```python
from build123d import *

# Parameters (mm, degrees)
EXTRUDE_1_DEPTH     = 8
SKETCH_2_W          = 51
SKETCH_2_H          = 5
EXTRUDE_2_DEPTH     = 28.7
SKETCH_3_R          = 17.5
CUT_EXTRUDE_1_DEPTH = 2
CUT_EXTRUDE_2_REACH = 82.708
SKETCH_4_R          = 1.25
SKETCH_5_R          = 1.5
CUT_EXTRUDE_3_DEPTH = 5


with BuildPart() as part:
    # 스케치1 → 보스-돌출1 (new body)
    with BuildSketch(Plane.XY):
        with BuildLine():
            Line((0, 0), (0, 54.5))
            Line((0, 54.5), (51, 54.5))
            Line((51, 54.5), (51, 0))
            ThreePointArc((51, 0), (25.5, -25.5), (0, 0))
        make_face()
    extrude(amount=EXTRUDE_1_DEPTH)

    # 스케치2 → 보스-돌출2 (add)
    with BuildSketch(Plane(origin=(0, 0, 0), x_dir=(-1, 0, 0), z_dir=(0, 0, -1))):
        with Locations((-25.5, 52)):
            Rectangle(SKETCH_2_W, SKETCH_2_H)
    extrude(amount=EXTRUDE_2_DEPTH)

    # 스케치3 → 컷-돌출1 (cut)
    with BuildSketch(Plane(origin=(0, 0, 0), x_dir=(-1, 0, 0), z_dir=(0, 0, -1))):
        with Locations((-25.5, 0)):
            Circle(SKETCH_3_R)
    extrude(amount=-CUT_EXTRUDE_1_DEPTH, mode=Mode.SUBTRACT)

    # 스케치4 → 컷-돌출2 (cut, up to next)
    with BuildSketch(Plane(origin=(0, 0, 2), x_dir=(-1, 0, 0), z_dir=(0, 0, -1)), mode=Mode.PRIVATE) as cut_extrude_2_sk1:
        with Locations((-25.5, 13.75)):
            Circle(SKETCH_4_R)
    cut_extrude_2_tool1 = extrude(cut_extrude_2_sk1.sketch, amount=-CUT_EXTRUDE_2_REACH, mode=Mode.PRIVATE) & part.part
    # 스케치4 → 컷-돌출2 (cut, up to next)
    with BuildSketch(Plane(origin=(0, 0, 2), x_dir=(-1, 0, 0), z_dir=(0, 0, -1)), mode=Mode.PRIVATE) as cut_extrude_2_sk2:
        with Locations((-13.592150698, 6.875)):
            Circle(SKETCH_4_R)
    cut_extrude_2_tool2 = extrude(cut_extrude_2_sk2.sketch, amount=-CUT_EXTRUDE_2_REACH, mode=Mode.PRIVATE) & part.part
    # 스케치4 → 컷-돌출2 (cut, up to next)
    with BuildSketch(Plane(origin=(0, 0, 2), x_dir=(-1, 0, 0), z_dir=(0, 0, -1)), mode=Mode.PRIVATE) as cut_extrude_2_sk3:
        with Locations((-13.592150698, -6.875)):
            Circle(SKETCH_4_R)
    cut_extrude_2_tool3 = extrude(cut_extrude_2_sk3.sketch, amount=-CUT_EXTRUDE_2_REACH, mode=Mode.PRIVATE) & part.part
    # 스케치4 → 컷-돌출2 (cut, up to next)
    with BuildSketch(Plane(origin=(0, 0, 2), x_dir=(-1, 0, 0), z_dir=(0, 0, -1)), mode=Mode.PRIVATE) as cut_extrude_2_sk4:
        with Locations((-25.5, -13.75)):
            Circle(SKETCH_4_R)
    cut_extrude_2_tool4 = extrude(cut_extrude_2_sk4.sketch, amount=-CUT_EXTRUDE_2_REACH, mode=Mode.PRIVATE) & part.part
    # 스케치4 → 컷-돌출2 (cut, up to next)
    with BuildSketch(Plane(origin=(0, 0, 2), x_dir=(-1, 0, 0), z_dir=(0, 0, -1)), mode=Mode.PRIVATE) as cut_extrude_2_sk5:
        with Locations((-37.407849302, -6.875)):
            Circle(SKETCH_4_R)
    cut_extrude_2_tool5 = extrude(cut_extrude_2_sk5.sketch, amount=-CUT_EXTRUDE_2_REACH, mode=Mode.PRIVATE) & part.part
    # 스케치4 → 컷-돌출2 (cut, up to next)
    with BuildSketch(Plane(origin=(0, 0, 2), x_dir=(-1, 0, 0), z_dir=(0, 0, -1)), mode=Mode.PRIVATE) as cut_extrude_2_sk6:
        with Locations((-37.407849302, 6.875)):
            Circle(SKETCH_4_R)
    cut_extrude_2_tool6 = extrude(cut_extrude_2_sk6.sketch, amount=-CUT_EXTRUDE_2_REACH, mode=Mode.PRIVATE) & part.part
    add(cut_extrude_2_tool1.solids().sort_by_distance((25.5, 13.75, 2))[0], mode=Mode.SUBTRACT)
    add(cut_extrude_2_tool2.solids().sort_by_distance((13.592151, 6.875, 2))[0], mode=Mode.SUBTRACT)
    add(cut_extrude_2_tool3.solids().sort_by_distance((13.592151, -6.875, 2))[0], mode=Mode.SUBTRACT)
    add(cut_extrude_2_tool4.solids().sort_by_distance((25.5, -13.75, 2))[0], mode=Mode.SUBTRACT)
    add(cut_extrude_2_tool5.solids().sort_by_distance((37.407849, -6.875, 2))[0], mode=Mode.SUBTRACT)
    add(cut_extrude_2_tool6.solids().sort_by_distance((37.407849, 6.875, 2))[0], mode=Mode.SUBTRACT)

    # 스케치5 → 컷-돌출3 (cut)
    with BuildSketch(Plane(origin=(0, 54.5, 0), x_dir=(1, 0, 0), z_dir=(0, 1, 0))):
        with Locations(Location((15.5, 22, 0), (0, 0, 270))):
            Circle(SKETCH_5_R)
        with Locations(Location((35.5, 22, 0), (0, 0, 270))):
            Circle(SKETCH_5_R)
        with Locations(Location((35.5, 2, 0), (0, 0, 270))):
            Circle(SKETCH_5_R)
        with Locations(Location((15.5, 2, 0), (0, 0, 270))):
            Circle(SKETCH_5_R)
    extrude(amount=-CUT_EXTRUDE_3_DEPTH, mode=Mode.SUBTRACT)


solid = part.part
```
For this review, take the finished solid that the model builds, in its own axes (mm). A direction names the side the tool comes from. Coordinates: 2 decimals unless noted, no trailing zeros. Write each loop counter-clockwise with the first axis right and the second up, starting at its lowest first coordinate (ties: lowest second). Pieces come first, ordered by that corner, then holes. Notation, with made-up numbers: (62, 48) - (112, 48) arc R18 cw to (112, 64) - close; hole circle Ø1 at (-8, -9.75). An arc over 180 degrees is marked (long way). Answer in a Markdown table with one row per item. Add a question column.
Q1. We need section D-D, the plane x = 20. State the section outline as (y, z) points.
Q2. We need section B-B, the plane z = -2. State the section outline as (x, y) points.
Q3. For P1, Ø2.5, axis at x = 35.5, z = -22, coming from the -Y side (3 decimals); P2, Ø1.5, axis at x = 7.5, y = 32, coming from the -Z side; P3, Ø1, axis at x = 15.5, z = -7, coming from the -Y side, all flat-tipped, find the tip position at first contact; note any pin that passes through.
Q4. We need section A-A, the plane x = 25.5. State the section outline as (y, z) points, and give its area (4 significant figures).
Q5. Tool access review of faces 4 (the flat face through (26, 21, 0)), 5 (the cylindrical face through (39.387, -10.648, 0.986)), 6 (the cylindrical face through (16.765, 52.035, -1.194)): name each direction out of +Z, -Z, +X, -X, +Y, -Y from which nothing blocks a thin tool from reaching the whole face with its end or side.
Q6. Draft analysis for pull direction X (two halves, no side actions). For faces 1 (the cylindrical face through (38.4, 6.114, 4.958)), 2 (the flat face through (26, 49.5, -14)), 3 (the cylindrical face through (26.061, -25.494, 3.944)), state which applies: +X half, -X half, draft (parallel to the pull), parting line (faces both ways), or undercut.
Q7. We need section C-C, the plane y = -13.75. State the section outline as (x, z) points.
Q8. For probe 1 along X at (y, z) = (-7, 6.5); probe 2 along Y at (x, z) = (20, -27); probe 3 along Z at (x, y) = (34.5, 11.5), list the stretches that pass through material, from the lowest coordinate up.
Answer list:
| question | item | result |
|---|---|---|
| 1 | outline | (-24.9, 0) - (-16.61, 0) - (-16.61, 2) - (16.61, 2) - (16.61, 0) - (49.5, 0) - (49.5, -28.7) - (54.5, -28.7) - (54.5, 8) - (-24.9, 8) - close |
| 2 | outline | (0, 49.5) - (14, 49.5) - (14, 54.5) - (0, 54.5) - close; (17, 49.5) - (34, 49.5) - (34, 54.5) - (17, 54.5) - close; (37, 49.5) - (51, 49.5) - (51, 54.5) - (37, 54.5) - close |
| 3 | P1 | passes through |
| 3 | P2 | stops at z = 0 |
| 3 | P3 | stops at y = 49.5 |
| 4 | outline | (-25.5, 0) - (-17.5, 0) - (-17.5, 2) - (-15, 2) - (-15, 8) - (-25.5, 8) - close; (-12.5, 2) - (12.5, 2) - (12.5, 8) - (-12.5, 8) - close; (15, 2) - (17.5, 2) - (17.5, 0) - (49.5, 0) - (49.5, -28.7) - (54.5, -28.7) - (54.5, 8) - (15, 8) - close |
| 4 | area | 683.5 mm2 |
| 5 | face 4 | -Z, +X, -X, -Y |
| 5 | face 5 | -Z |
| 5 | face 6 | +Y, -Y |
| 6 | face 1 | undercut |
| 6 | face 2 | draft |
| 6 | face 3 | parting line |
| 7 | outline | (4.02, 0) - (14.67, 0) - (14.67, 2) - (24.25, 2) - (24.25, 8) - (4.02, 8) - close; (26.75, 2) - (36.33, 2) - (36.33, 0) - (46.98, 0) - (46.98, 8) - (26.75, 8) - close |
| 8 | probe 1 | x = 0.98 to 12.35, 14.84 to 36.16, 38.65 to 50.02 |
| 8 | probe 2 | y = 49.5 to 54.5 |
| 8 | probe 3 | z = 2 to 8 |
